from build123d import *

# Parameters (mm, degrees)
BOSS_EXTRUDE1_DEPTH = 60
BOSS_EXTRUDE2_DEPTH = 0.5
CUT_EXTRUDE1_DEPTH  = 2
CUT_EXTRUDE2_REACH  = 15
SKETCH6_R           = 2
CUT_EXTRUDE3_REACH  = 4
SKETCH7_R           = 2
SKETCH8_R           = 2
CUT_EXTRUDE4_DEPTH  = 2


with BuildPart() as part:
    # Sketch1 → Boss-Extrude1 (new body)
    with BuildSketch(Plane.XY):
        Polygon((0, 0), (-11, 0), (-11, 38), (-13, 38), (-13, -2), (0, -2), align=None)
    extrude(amount=BOSS_EXTRUDE1_DEPTH)

    # Sketch4 → Boss-Extrude2 (add, symmetric)
    with BuildSketch(Plane.XY.offset(30)):
        Polygon((-11, 20), (-1, 0), (-11, 0), align=None)
    extrude(amount=BOSS_EXTRUDE2_DEPTH, both=True)

    # Sketch5 → Cut-Extrude1 (cut)
    with BuildSketch(Plane(origin=(0, 0, 0), x_dir=(1, 0, 0), z_dir=(0, 1, 0))):
        with BuildLine():
            Line((-3, -5), (-3, -10))
            ThreePointArc((-3, -10), (-6, -13), (-9, -10))
            Line((-9, -10), (-9, -5))
            ThreePointArc((-9, -5), (-6, -2), (-3, -5))
        make_face()
    cut_extrude1 = extrude(amount=-CUT_EXTRUDE1_DEPTH, mode=Mode.SUBTRACT)

    # Mirror1: Cut-Extrude1 across plane
    add(cut_extrude1.mirror(Plane.XY.offset(30)), mode=Mode.SUBTRACT)

    # Sketch6 → Cut-Extrude2 (cut, up to next)
    with BuildSketch(Plane(origin=(-13, 0, 0), x_dir=(0, 0, -1), z_dir=(1, 0, 0)), mode=Mode.PRIVATE) as cut_extrude2_sk1:
        with Locations((-50, 31)):
            Circle(SKETCH6_R)
    cut_extrude2_tool1 = extrude(cut_extrude2_sk1.sketch, amount=CUT_EXTRUDE2_REACH, mode=Mode.PRIVATE) & part.part
    add(cut_extrude2_tool1.solids().sort_by_distance((-13, 31, 50))[0], mode=Mode.SUBTRACT)
    # Sketch6 → Cut-Extrude2 (cut, up to next)
    with BuildSketch(Plane(origin=(-13, 0, 0), x_dir=(0, 0, -1), z_dir=(1, 0, 0)), mode=Mode.PRIVATE) as cut_extrude2_sk2:
        with Locations((-10, 31)):
            Circle(SKETCH6_R)
    cut_extrude2_tool2 = extrude(cut_extrude2_sk2.sketch, amount=CUT_EXTRUDE2_REACH, mode=Mode.PRIVATE) & part.part
    add(cut_extrude2_tool2.solids().sort_by_distance((-13, 31, 10))[0], mode=Mode.SUBTRACT)

    # Sketch7 → Cut-Extrude3 (cut, up to next)
    with BuildSketch(Plane(origin=(-11, 0, 0), x_dir=(0, 0, -1), z_dir=(1, 0, 0)), mode=Mode.PRIVATE) as cut_extrude3_sk1:
        with Locations((-30, 28)):
            Circle(SKETCH7_R)
    cut_extrude3_tool1 = extrude(cut_extrude3_sk1.sketch, amount=-CUT_EXTRUDE3_REACH, mode=Mode.PRIVATE) & part.part
    add(cut_extrude3_tool1.solids().sort_by_distance((-11, 28, 30))[0], mode=Mode.SUBTRACT)

    # Sketch8 → Cut-Extrude4 (cut)
    with BuildSketch(Plane(origin=(0, 0, 0), x_dir=(1, 0, 0), z_dir=(0, 1, 0))):
        with Locations((-5, -37.5)):
            Circle(SKETCH8_R)
    cut_extrude4 = extrude(amount=-CUT_EXTRUDE4_DEPTH, mode=Mode.SUBTRACT)

    # Mirror2: Cut-Extrude4 across plane
    add(cut_extrude4.mirror(Plane.XY.offset(30)), mode=Mode.SUBTRACT)


solid = part.part
Verification items for the finished model (mm, model axes). A direction names the side the tool comes from. Round coordinates to 2 decimals unless told otherwise and drop trailing zeros. Loops run counter-clockwise (first coordinate to the right, second up) from the corner with the lowest first, then second, coordinate; pieces in that order, holes last. Notation, with made-up numbers: (58.5, 38.25) - (98.5, 38.25) arc R10 ccw to (98.5, 52.25) - close; hole circle Ø9 at (-23.5, 30). An arc over 180 degrees is marked (long way). Answer in a Markdown table with one row per item. Add a question column.
Q1. Section check C-C on y = 8.5. Enter the section's corners in (x, z), plus the area to 3 significant figures.
Q2. Gauge pin test, flat ends, axial feed: pin 1 (1 mm diameter, centred on x = -8.5, z = 17.5, fed in from +Y); pin 2 (5 mm diameter, centred on y = 31, z = 50, fed in from +X); pin 3 (3 mm diameter, centred on x = -8, y = 9.5, fed in from -Z). Record the tip position at first contact, or that the pin passes through.
Q3. Tool access check on faces 4 (the face through (-9, -1, 8)), 5 (the face through (-11, 23, 30)), 6 (the face through (-8, 6, 30.5)). Record the directions out of +Z, -Z, +X, -X, +Y, -Y that give a thin tool (end or side, any length) a straight path to the whole face; none if there is none.
Q4. Material ranges on line 1 (Z direction, x = -11.9, y = 31); line 2 (Y direction, x = -11.6, z = 10); line 3 (Z direction, x = -5, y = -0.8), recorded low to high.
Q5. Section check B-B on x = -11.75. Enter the section's corners in (y, z).
Q6. Section check A-A on z = 37.5. Enter the section's corners in (x, y), plus the area to 3 significant figures.
Q7. Section check D-D on x = -5. Enter the section's corners in (y, z).
Q8. Release check for a two-part mould opening along X. For faces 1 (the face through (-11.3, 15.1, 0)), 2 (the face through (-5.434, -0.986, 39.452)), 3 (the face through (-6, 10, 30)) record: pulls with the +X half, pulls with the -X half, needs draft (parallel to the pull), parting line crosses it, or undercut.
Found:
| question | item | result |
|---|---|---|
| 1 | outline | (-13, 0) - (-11, 0) - (-11, 29.5) - (-5.25, 29.5) - (-5.25, 30.5) - (-11, 30.5) - (-11, 60) - (-13, 60) - close |
| 1 | area | 126 mm² |
| 2 | pin 1 | stops at y = 0 |
| 2 | pin 2 | stops at x = -11 |
| 2 | pin 3 | stops at z = 29.5 |
| 3 | face 4 | +Y, -Y |
| 3 | face 5 | +X, +Y |
| 3 | face 6 | +Z, +X, +Y |
| 4 | line 1 | z = 0 to 8, 12 to 48, 52 to 60 |
| 4 | line 2 | y = -2 to 29, 33 to 38 |
| 4 | line 3 | z = 0 to 2.17, 12.83 to 20.5, 24.5 to 35.5, 39.5 to 47.17, 57.83 to 60 |
| 5 | outline | (-2, 0) - (38, 0) - (38, 60) - (-2, 60) - close; hole circle Ø4 at (28, 30); hole circle Ø4 at (31, 10); hole circle Ø4 at (31, 50) |
| 6 | outline | (-13, -2) - (-7, -2) - (-7, 0) - (-11, 0) - (-11, 38) - (-13, 38) - close; (-3, -2) - (0, -2) - (0, 0) - (-3, 0) - close |
| 6 | area | 94.0 mm² |
| 7 | outline | (-2, 0) - (0, 0) - (0, 2.17) - (-2, 2.17) - close; (-2, 12.83) - (0, 12.83) - (0, 20.5) - (-2, 20.5) - close; (-2, 24.5) - (0, 24.5) - (0, 29.5) - (8, 29.5) - (8, 30.5) - (0, 30.5) - (0, 35.5) - (-2, 35.5) - close; (-2, 39.5) - (0, 39.5) - (0, 47.17) - (-2, 47.17) - close; (-2, 57.83) - (0, 57.83) - (0, 60) - (-2, 60) - close |
| 8 | face 1 | needs draft |
| 8 | face 2 | undercut |
| 8 | face 3 | pulls with the +X half |
